```python
from build123d import *

# Parameters (mm, degrees)
SKETCH1_W                = 66.294
SKETCH1_H                = 112.776
BOSS_EXTRUDE1_DEPTH      = 3.048
SKETCH2_W                = 66.294
SKETCH2_H                = 112.776
SKETCH2_W_2              = 60
SKETCH2_H_2              = 106.68
BOSS_EXTRUDE2_DEPTH      = 31.75
SKETCH3_W                = 60
SKETCH3_H                = 8.89
BOSS_EXTRUDE3_DEPTH      = 3.048
SKETCH6_W                = 106.68
SKETCH6_H                = 31.75
CUT_EXTRUDE1_DEPTH       = 3.302
M3_CLEARANCE_HOLE1_D     = 3.4
M3_CLEARANCE_HOLE1_DEPTH = 3.048
CUT_EXTRUDE4_REACH       = 124.589
SKETCH12_W               = 40.894
SKETCH12_H               = 20.32
SKETCH13_W               = 17.78
SKETCH13_H               = 5.08
BOSS_EXTRUDE4_DEPTH      = 5.08
SKETCH14_W               = 17.78
SKETCH14_H               = 2.54
BOSS_EXTRUDE6_DEPTH      = 5.08


with BuildPart() as part:
    # Sketch1 → Boss-Extrude1 (new body)
    with BuildSketch(Plane(origin=(0, 0, 0), x_dir=(1, 0, 0), z_dir=(0, 1, 0))):
        Rectangle(SKETCH1_W, SKETCH1_H)
    extrude(amount=BOSS_EXTRUDE1_DEPTH)

    # Sketch2 → Boss-Extrude2 (add)
    with BuildSketch(Plane(origin=(0, 3.048, 0), x_dir=(1, 0, 0), z_dir=(0, 1, 0))):
        Rectangle(SKETCH2_W, SKETCH2_H)
        Rectangle(SKETCH2_W_2, SKETCH2_H_2, mode=Mode.SUBTRACT)
    extrude(amount=BOSS_EXTRUDE2_DEPTH)

    # Sketch3 → Boss-Extrude3 (add)
    with BuildSketch(Plane(origin=(0, 34.798, 0), x_dir=(1, 0, 0), z_dir=(0, 1, 0))):
        with Locations((0, 48.895)):
            Rectangle(SKETCH3_W, SKETCH3_H)
        with Locations((0, -48.895)):
            Rectangle(SKETCH3_W, SKETCH3_H)
    extrude(amount=-BOSS_EXTRUDE3_DEPTH)

    # Sketch6 → Cut-Extrude1 (cut)
    with BuildSketch(Plane(origin=(33.147, 0, 0), x_dir=(0, 0, -1), z_dir=(1, 0, 0))):
        with Locations((0, 18.923)):
            Rectangle(SKETCH6_W, SKETCH6_H)
    extrude(amount=-CUT_EXTRUDE1_DEPTH, mode=Mode.SUBTRACT)

    # M3 Clearance Hole1
    with Locations(Plane(origin=(-20.447, 34.798, -50.038), x_dir=(0, 0, 1), z_dir=(0, 1, 0))):
        with Locations((0, 0), (0, 40.894), (100.076, 0), (100.076, 40.894)):
            Hole(M3_CLEARANCE_HOLE1_D / 2, depth=M3_CLEARANCE_HOLE1_DEPTH)

    # Sketch12 → Cut-Extrude4 (cut, up to next)
    with BuildSketch(Plane(origin=(0, 0, -56.388), x_dir=(-1, 0, 0), z_dir=(0, 0, -1)), mode=Mode.PRIVATE) as cut_extrude4_sk1:
        with Locations((0, 13.208)):
            Rectangle(SKETCH12_W, SKETCH12_H)
    cut_extrude4_tool1 = extrude(cut_extrude4_sk1.sketch, amount=-CUT_EXTRUDE4_REACH, mode=Mode.PRIVATE) & part.part
    add(cut_extrude4_tool1.solids().sort_by_distance((0, 13.208, -56.388))[0], mode=Mode.SUBTRACT)

    # Sketch13 → Boss-Extrude4 (add)
    with BuildSketch(Plane.XZ):
        with Locations((0, 12.7)):
            Rectangle(SKETCH13_W, SKETCH13_H)
        with Locations((0, -12.7)):
            Rectangle(SKETCH13_W, SKETCH13_H)
    extrude(amount=BOSS_EXTRUDE4_DEPTH)

    # Sketch14 → Boss-Extrude6 (add)
    with BuildSketch(Plane(origin=(0, 0, 10.16), x_dir=(-1, 0, 0), z_dir=(0, 0, -1))):
        with Locations((0, -3.81)):
            Rectangle(SKETCH14_W, SKETCH14_H)
    boss_extrude6 = extrude(amount=BOSS_EXTRUDE6_DEPTH)

    # Mirror2: Boss-Extrude6 across plane
    add(boss_extrude6.mirror(Plane(origin=(0, 0, 0), x_dir=(1, 0, 0), z_dir=(0, 0, -1))))


solid = part.part
```
Model file for the job. Use its own axes, mm. A direction names the side the tool comes from. Coordinates: 2 decimals unless noted, no trailing zeros. Write each loop counter-clockwise with the first axis right and the second up, starting at its lowest first coordinate (ties: lowest second). Pieces come first, ordered by that corner, then holes. Notation, with made-up numbers: (34.25, 57) - (65.25, 57) arc R26 ccw to (65.25, 78) - close; hole circle Ø2 at (-29, 84). An arc over 180 degrees is marked (long way). One line per item, written item: value. Start each with the question number.
1. Slice it at C-C (y = 29). Write the cut outline in (x, z), plus the area to 3 significant figures.
2. Tool access for faces 5 (the flat face through (0, -1, -10.16)), 6 (the flat face through (0, -3, 15.24)), 7 (the flat face through (0, -4, 5.08)): list every direction of +Z, -Z, +X, -X, +Y, -Y with a clear straight run to the whole face (end or side of a thin tool).
3. Mould opens along X. For faces 1 (the flat face through (20.447, 13, -55)), 2 (the flat face through (0, 23.368, -55)), 3 (the flat face through (0, -2.54, -8)), 4 (the flat face through (29.845, 33, 49)) say: released by +X, released by -X, zero draft, split by the parting line, or undercut.
4. Slice it at B-B (y = 11.5). Write the cut outline in (x, z).
5. Probe line 1 (Y direction, x = 21, z = 45.5); line 2 (Z direction, x = 26, y = 9); line 3 (Y direction, x = -3, z = 8). List the from-to ranges inside material, lowest first. Write a range as from..to.
6. Slice it at D-D (x = -14.5). Write the cut outline in (y, z), plus the area to 3 significant figures.
7. Slice it at A-A (x = -3.5). Write the cut outline in (y, z).
8. Flat gauge pins, fed straight in: pin 1 (5 mm diameter, centred on x = 23.5, z = 19.5, fed in from +Y); pin 2 (8 mm diameter, centred on x = 6, z = -44.5, fed in from -Y); pin 3 (1 mm diameter, centred on y = 16, z = 6, fed in from +X). Where does each tip first touch, or does it go through?
Answers below:
1. outline: (-33.15, -56.39) - (33.15, -56.39) - (33.15, -53.34) - (-30, -53.34) - (-30, 53.34) - (33.15, 53.34) - (33.15, 56.39) - (-33.15, 56.39) - close
1. area: 740 mm^2
2. face 5: +X, -X
2. face 6: +Z, +X, -X, -Y
2. face 7: +X, -X, -Y
3. face 1: undercut
3. face 2: undercut
3. face 3: zero draft
3. face 4: released by +X
4. outline: (-33.15, -56.39) - (-20.45, -56.39) - (-20.45, -53.34) - (-30, -53.34) - (-30, 53.34) - (33.15, 53.34) - (33.15, 56.39) - (-33.15, 56.39) - close; (20.45, -56.39) - (33.15, -56.39) - (33.15, -53.34) - (20.45, -53.34) - close
5. line 1: y = 0..3.05, 31.75..34.8
5. line 2: z = -56.39..-53.34, 53.34..56.39
5. line 3: y = -5.08..-2.54, 0..3.05
6. outline: (0, -56.39) - (3.05, -56.39) - (3.05, 53.34) - (31.75, 53.34) - (31.75, 44.45) - (34.8, 44.45) - (34.8, 56.39) - (0, 56.39) - close; (23.37, -56.39) - (34.8, -56.39) - (34.8, -44.45) - (31.75, -44.45) - (31.75, -53.34) - (23.37, -53.34) - close
6. area: 530 mm^2
7. outline: (-5.08, -15.24) - (0, -15.24) - (0, -56.39) - (3.05, -56.39) - (3.05, 53.34) - (31.75, 53.34) - (31.75, 44.45) - (34.8, 44.45) - (34.8, 56.39) - (0, 56.39) - (0, 15.24) - (-5.08, 15.24) - (-5.08, 5.08) - (-2.54, 5.08) - (-2.54, 10.16) - (0, 10.16) - (0, -10.16) - (-2.54, -10.16) - (-2.54, -5.08) - (-5.08, -5.08) - close; (23.37, -56.39) - (34.8, -56.39) - (34.8, -44.45) - (31.75, -44.45) - (31.75, -53.34) - (23.37, -53.34) - close
8. pin 1: stops at y = 3.05
8. pin 2: stops at y = 0
8. pin 3: stops at x = -30
